from build123d import *

# Parameters (mm, degrees)
SKETCH_W    = 23.713642
SKETCH_H    = 32.997763
PAD_DEPTH   = 15
FILLET_R    = 12
FILLET001_R = 10


with BuildPart() as part:
    # Sketch (on XZ_Plane of Origin) → Pad (new body)
    with BuildSketch(Plane.XZ):
        with Locations((3.5793, -3.187445)):
            Rectangle(SKETCH_W, SKETCH_H)
    extrude(amount=PAD_DEPTH)

    # Fillet
    fillet_edges = [part.edges().sort_by_distance(p)[0] for p in [
        (-8.277521, -7.5, -19.686327),
    ]]
    fillet(fillet_edges, radius=FILLET_R)

    # Fillet001
    fillet001_edges = [part.edges().sort_by_distance(p)[0] for p in [
        (3.5793, 0, 13.311436),
    ]]
    fillet(fillet001_edges, radius=FILLET001_R)


solid = part.part
Could you check a few things on this model? Use its own coordinates, in mm. Round coordinates to 2 decimals unless told otherwise and drop trailing zeros. Order: outer loops, then holes, each group sorted by start corner. A loop starts at its lowest first (then second) coordinate and runs counter-clockwise, first axis right, second up. Notation, with made-up numbers: M 73,-24 L 121,-24 A14 cw 121,-6 Z; hole C 14.5,41.25 d7. An arc over 180 degrees is marked long. One line per item, written item: value.
(1) Imagine slicing it at C-C (z = -15). Write out the boundary of the cut face in (x, y).
Ans:
outline: M -5.79,-15 L 15.44,-15 L 15.44,0 L -5.79,0 Z
(2) I'm going to push flat-ended pins straight in: P1, Ø5, axis at x = 7.5, y = -3, coming from the +Z side; P2, Ø2, axis at x = 4.5, y = -5, coming from the +Z side; P3, Ø3, axis at x = -0.5, y = -11.5, coming from the -Z side. Where does each tip first touch, or does it pass through?
Ans:
P1: stops at z = 12.24
P2: stops at z = 12.48
P3: stops at z = -19.37
(3) Imagine slicing it at B-B (x = 8.25). Write out the boundary of the cut face in (y, z), and give its area (3 significant figures).
Ans:
outline: M -15,-19.69 L 0,-19.69 L 0,3.31 A10 ccw -10,13.31 L -15,13.31 Z
area: 474 mm^2
(4) I need wall thicknesses on line 1 along Z through (x, y) = (9, -4); line 2 along Y through (x, z) = (2.5, 5); line 3 along Z through (x, y) = (4.5, -6.5). Which ranges of each line are inside material? Lowest first, please. Write a range as from..to.
Ans:
line 1: z = -19.69..11.31
line 2: y = -15..-0.14
line 3: z = -19.69..12.68
(5) Imagine slicing it at D-D (z = 10). Write out the boundary of the cut face in (x, y), and give its area (3 significant figures).
Ans:
outline: M -8.28,-15 L 15.44,-15 L 15.44,-2.57 L -8.28,-2.57 Z
area: 295 mm^2
(6) Imagine slicing it at A-A (y = -11). Write out the boundary of the cut face in (x, z).
Ans:
outline: M -8.28,-7.69 A12 ccw 3.72,-19.69 L 15.44,-19.69 L 15.44,13.31 L -8.28,13.31 Z
